Source: three-view drawing plus pictorial views. Frame: mm from the lowest corner of the part. A direction names the side the tool comes from. Give positions to 0.01 mm unless a question says otherwise; leave off trailing zeros. Loops run counter-clockwise (first coordinate to the right, second up) from the corner with the lowest first, then second, coordinate; pieces in that order, holes last. Notation, with made-up numbers: M -20.5,16 L -10.5,16 A30 ccw -10.5,41 Z; hole C 28.5,36.25 d11. An arc over 180 degrees is marked long. Answer as a JSON object with one key per item and string values. Group by question number.
1) Draft query along X for the marked faces 3, 4 and 5. Return one class per face: +X half, -X half, draft (parallel to the pull), parting line (faces both ways), or undercut.
2) Section query C-C on y = 8. Return loops of the section in (x, z).
3) Section query A-A on x = 8. Return loops of the section in (y, z).
4) Section query D-D on z = 24.5. Return loops of the section in (x, y), plus the area to 3 significant figures.
5) Section query B-B on z = 5. Return loops of the section in (x, y).
6) Ray query, L1, parallel to Z at x = 6.5, y = 2; L2, parallel to X at y = 3.5, z = 7.5 (1 decimal); L3, parallel to X at y = 6.25, z = 7. Return the intervals inside material, ascending.
7) First-contact query: P1, Ø1, axis at y = 11, z = 16, coming from the +X side; P2, Ø1, axis at y = 9, z = 9.5, coming from the -X side; P3, Ø1.5, axis at x = 13.5, z = 26.5, coming from the +Y side. Flat tips, straight axial feed; report the tip coordinate or a pass-through.
8) Access query for the marked faces 1 and 2. Directions: +Z, -Z, +X, -X, +Y, -Y. A direction counts if a zero-diameter tool reaches every point of the face in a straight line with its end or side. Return the directions, or none.
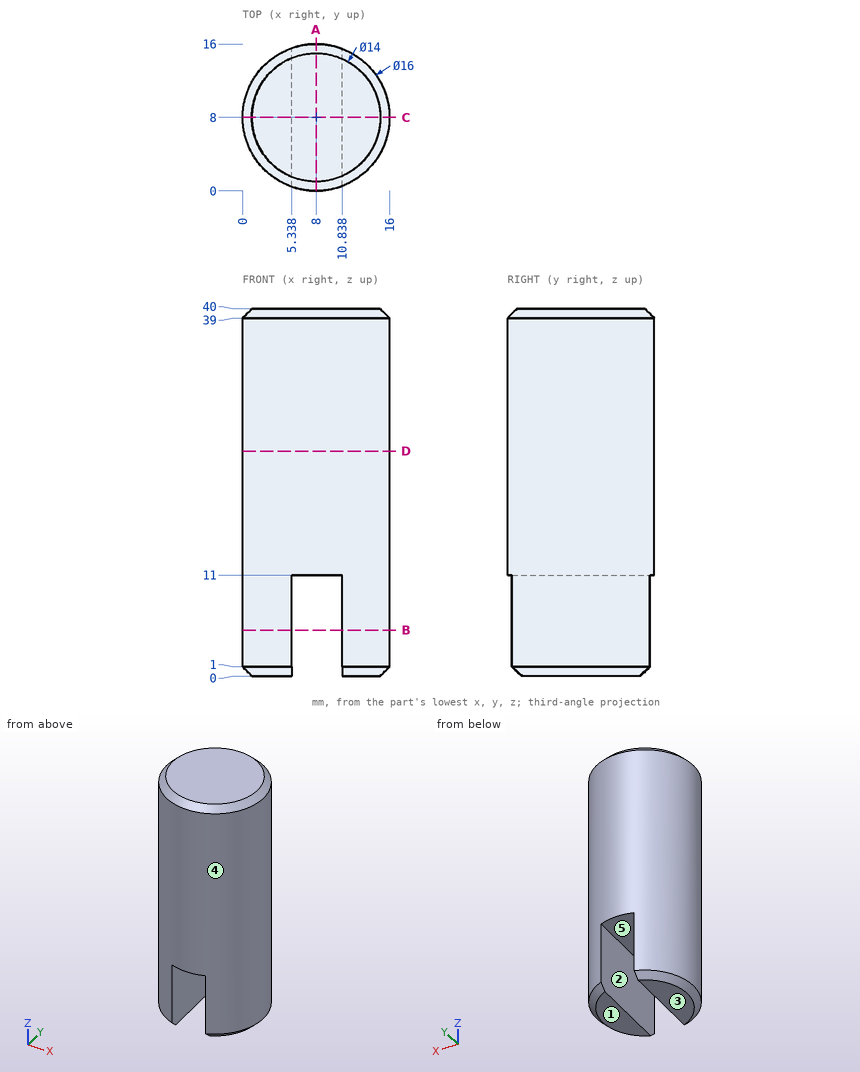
Output:
{
 "1": {"face 3": "draft", "face 4": "parting line", "face 5": "undercut"},
 "2": {"outline": "M 0,1 L 1,0 L 5.34,0 L 5.34,11 L 10.84,11 L 10.84,0 L 15,0 L 16,1 L 16,39 L 15,40 L 1,40 L 0,39 Z"},
 "3": {"outline": "M 0,11 L 16,11 L 16,39 L 15,40 L 1,40 L 0,39 Z"},
 "4": {"outline": "C 8,8 d16", "area": "201 mm^2"},
 "5": {"outline": "M 5.34,0.46 L 5.34,15.54 A8 ccw Z; M 10.84,0.52 A8 ccw 10.84,15.48 Z"},
 "6": {"L1": "z = 11 to 40", "L2": "x = 1.4 to 5.3, 10.8 to 14.6", "L3": "x = 0.19 to 5.34, 10.84 to 15.81"},
 "7": {"P1": "stops at x = 15.6", "P2": "stops at x = 0.02", "P3": "stops at y = 14.44"},
 "8": {"face 1": "-Z, +X, -X, +Y, -Y", "face 2": "-Z, +Y, -Y"}
}
